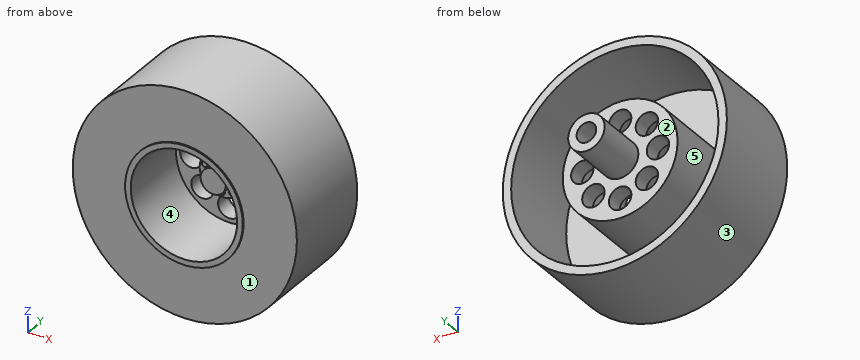
from build123d import *

# Parameters (mm, degrees)
F0_R      = 20
F1_DEPTH  = 17
F2_R      = 18.5
F3_DEPTH  = 15.5
F4_R      = 10.25
F5_DEPTH  = 14
F6_R      = 9.5
F7_DEPTH  = 12.5
F8_R      = 10.5
F8_R_2    = 9.5
F9_DEPTH  = 0.25
F10_R     = 2
F11_DEPTH = 5
F10_R_2   = 3.25
F12_DEPTH = 9.5
F13_R     = 1.75
F14_DEPTH = 9
F15_R     = 4
F16_DEPTH = 2
F17_R     = 0.5
F18_DEPTH = 0.25
F17_R_2   = 2.25
F19_DEPTH = 2.5


with BuildPart() as f1:
    # F0 (on Front) → F1 (new body)
    with BuildSketch(Plane.XZ):
        Circle(F0_R)
    extrude(amount=-F1_DEPTH)

    # F2 (on face) → F3 (cut)
    with BuildSketch(Plane(origin=(0, 17, 0), x_dir=(-1, 0, 0), z_dir=(0, 1, 0))):
        Circle(F2_R)
    extrude(amount=-F3_DEPTH, mode=Mode.SUBTRACT)

    # F4 (on face) → F5 (join)
    with BuildSketch(Plane(origin=(0, 1.5, 0), x_dir=(-1, 0, 0), z_dir=(0, 1, 0))):
        Circle(F4_R)
    extrude(amount=F5_DEPTH)

    # F6 (on face) → F7 (cut)
    with BuildSketch(Plane.XZ):
        Circle(F6_R)
    extrude(amount=-F7_DEPTH, mode=Mode.SUBTRACT)

    # F8 (on face) → F9 (join)
    with BuildSketch(Plane.XZ):
        Circle(F8_R)
        Circle(F8_R_2, mode=Mode.SUBTRACT)
    extrude(amount=F9_DEPTH)

    # F10 (on face) → F11 (cut)
    with BuildSketch(Plane(origin=(0, 15.5, 0), x_dir=(-1, 0, 0), z_dir=(0, 1, 0))):
        with Locations((0, 6.75)):
            Circle(F10_R)
        with Locations((4.772970773, 4.772970773)):
            Circle(F10_R)
        with Locations((6.75, 0)):
            Circle(F10_R)
        with Locations((4.772970773, -4.772970773)):
            Circle(F10_R)
        with Locations((0, -6.75)):
            Circle(F10_R)
        with Locations((-4.772970773, -4.772970773)):
            Circle(F10_R)
        with Locations((-6.75, 0)):
            Circle(F10_R)
        with Locations((-4.772970773, 4.772970773)):
            Circle(F10_R)
    extrude(amount=-F11_DEPTH, mode=Mode.SUBTRACT)

    # F10 (on face) → F12 (join)
    with BuildSketch(Plane(origin=(0, 15.5, 0), x_dir=(-1, 0, 0), z_dir=(0, 1, 0))):
        Circle(F10_R_2)
    extrude(amount=F12_DEPTH)

    # F13 (on face) → F14 (cut)
    with BuildSketch(Plane(origin=(0, 25, 0), x_dir=(-1, 0, 0), z_dir=(0, 1, 0))):
        Circle(F13_R)
    extrude(amount=-F14_DEPTH, mode=Mode.SUBTRACT)

    # F15 (on face) → F16 (join)
    with BuildSketch(Plane.XZ.offset(-12.5)):
        Circle(F15_R)
    extrude(amount=F16_DEPTH)

    # F17 (on face) → F18 (join)
    with BuildSketch(Plane.XZ.offset(-10.5)):
        with Locations((-2.9720516134, 0.9656781074)):
            Circle(F17_R)
        with Locations((-1.8368289134, 2.5281781074)):
            Circle(F17_R)
        with Locations((1.8368289134, 2.5281781074)):
            Circle(F17_R)
        with Locations((0, 3.125)):
            Circle(F17_R)
        with Locations((2.9720516134, -0.9656781074)):
            Circle(F17_R)
        with Locations((1.8368289134, -2.5281781074)):
            Circle(F17_R)
        with Locations((2.9720516134, 0.9656781074)):
            Circle(F17_R)
        with Locations((0, -3.125)):
            Circle(F17_R)
        with Locations((-2.9720516134, -0.9656781074)):
            Circle(F17_R)
        with Locations((-1.8368289134, -2.5281781074)):
            Circle(F17_R)
    extrude(amount=F18_DEPTH)

    # F17 (on face) → F19 (join)
    with BuildSketch(Plane.XZ.offset(-10.5)):
        Circle(F17_R_2)
    extrude(amount=F19_DEPTH)


solid = f1.part
The model under review builds one solid part; all positions refer to its coordinate system, in mm. Face numbers are marked on the shaded views. A direction names the side the tool comes from. Coordinates: 2 decimals unless noted, no trailing zeros. Write each loop counter-clockwise with the first axis right and the second up, starting at its lowest first coordinate (ties: lowest second). Pieces come first, ordered by that corner, then holes. Notation, with made-up numbers: (8.25, 41) - (47.25, 41) arc R13 cw to (47.25, 47) - close; hole circle Ø2 at (25, 52.25). An arc over 180 degrees is marked (long way). Answer as CSV lines item,"result".
(1) Tool access review of the marked faces 4 and 5: name each direction out of +Z, -Z, +X, -X, +Y, -Y from which nothing blocks a thin tool from reaching the whole face with its end or side.
Data:
face 4,"-Y"
face 5,"+Y"
(2) We need section C-C (x = 0). Count the separate pieces of the cut face and the enclosed holes in it, plus the area to 4 significant figures.
Data:
separate pieces,"3"
enclosed holes,"0"
area,"190.5 mm2"
(3) We need section D-D (z = -13). Give the boundary of the cut face in (x, y).
Data:
outline,"(-15.2, 0) - (15.2, 0) - (15.2, 17) - (13.16, 17) - (13.16, 1.5) - (-13.16, 1.5) - (-13.16, 17) - (-15.2, 17) - close"
(4) For line 1 along Z through (x, y) = (0, 9.25); line 2 along Z through (x, y) = (0, 13.75); line 3 along Z through (x, y) = (8.5, 6.75), list the stretches that pass through material, from the lowest coordinate up. Write a range as [from, to].
Data:
line 1,"z = [-20, -18.5], [-10.25, -9.5], [-2.25, 2.25], [9.5, 10.25], [18.5, 20]"
line 2,"z = [-20, -18.5], [-10.25, -8.75], [-4.75, 4.75], [8.75, 10.25], [18.5, 20]"
line 3,"z = [-18.1, -16.43], [-5.73, -4.24], [4.24, 5.73], [16.43, 18.1]"
(5) Clearance check with flat-ended pins moving along their axes: pin 1 Ø1.1 at (x, z) = (-2, 3) entering from -Y; pin 2 Ø1.3 at (x, z) = (-0.5, -1) entering from -Y; pin 3 Ø6.5 at (x, z) = (0, 6.75) entering from +Y. State where each tip first meets the part, or that it passes through.
Data:
pin 1,"stops at y = 10.25"
pin 2,"stops at y = 8"
pin 3,"stops at y = 15.5"
(6) We need section B-B (y = 3.75). Give the boundary of the cut face in (x, z).
Data:
outline,"circle Ø40 at (0, 0); circle Ø20.5 at (0, 0); hole circle Ø37 at (0, 0); hole circle Ø19 at (0, 0)"
(7) We need section A-A (y = 12). Give the boundary of the cut face in (x, z).
Data:
outline,"circle Ø40 at (0, 0); circle Ø20.5 at (0, 0); circle Ø8 at (0, 0); hole circle Ø37 at (0, 0); hole circle Ø19 at (0, 0)"
(8) Mouldability with a two-part tool opening along X and no side actions: class the marked faces 1, 2 and 3 as pulls with the +X half, pulls with the -X half, needs draft (parallel to the pull), parting line crosses it, or undercut.
Data:
face 1,"needs draft"
face 2,"undercut"
face 3,"parting line crosses it"
